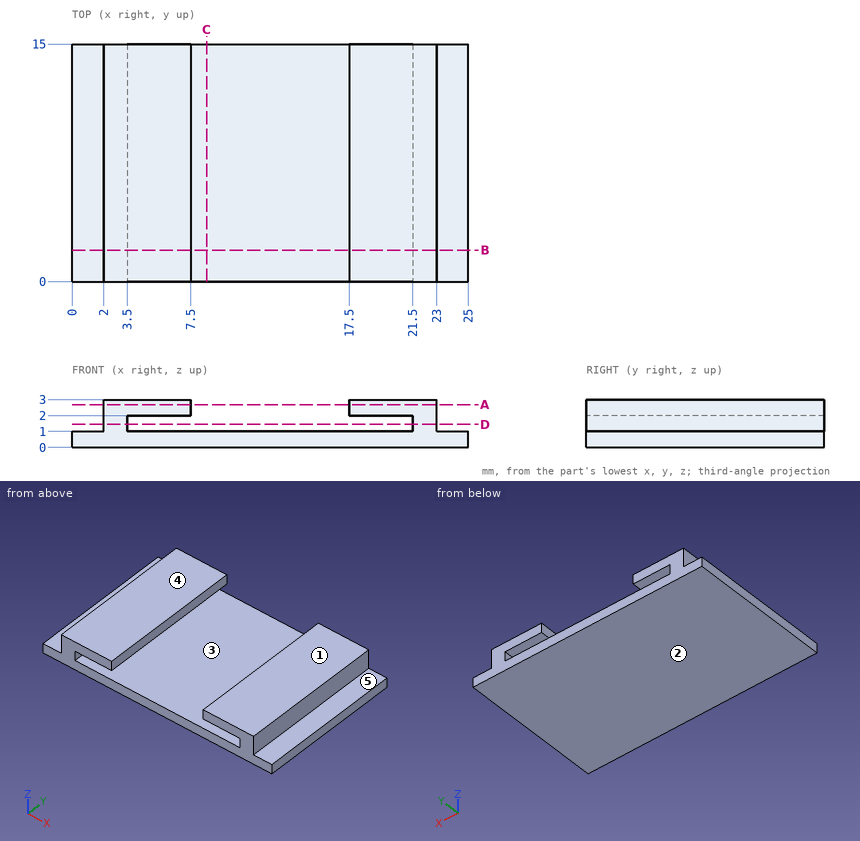
Drawing for the job (mm, zero at the part's lowest x, y, z). A direction names the side the tool comes from. Round coordinates to 2 decimals unless told otherwise and drop trailing zeros. Loops run counter-clockwise (first coordinate to the right, second up) from the corner with the lowest first, then second, coordinate; pieces in that order, holes last. Notation, with made-up numbers: (46.25, 8) - (51.25, 8) arc R9 ccw to (51.25, 17) - close; hole circle Ø9 at (86, 35). An arc over 180 degrees is marked (long way). Write each question's results on one line, items separated by ' | '.
(1) Mould opens along Z. For the marked faces 1, 2 and 3 say: released by +Z, released by -Z, zero draft, split by the parting line, or undercut.
Answer below:
face 1: released by +Z | face 2: released by -Z | face 3: undercut
(2) Pin check, flat tips, straight feed: pin 1 (6 mm diameter, centred on x = 11, y = 11, fed in from +Z); pin 2 (0.8 mm diameter, centred on y = 8.5, z = 1.5, fed in from -X); pin 3 (0.8 mm diameter, centred on y = 8.5, z = 1.5, fed in from +X). Stop position of each tip, or through.
Answer below:
pin 1: stops at z = 1 | pin 2: stops at x = 2 | pin 3: stops at x = 23
(3) Saw through at C-C, the plane x = 8.5. List the corners of the cut face in (y, z).
Answer below:
outline: (0, 0) - (15, 0) - (15, 1) - (0, 1) - close
(4) Saw through at A-A, the plane z = 2.7. List the corners of the cut face in (x, y).
Answer below:
outline: (2, 0) - (7.5, 0) - (7.5, 15) - (2, 15) - close; (17.5, 0) - (23, 0) - (23, 15) - (17.5, 15) - close
(5) Wall check: L1, parallel to X at y = 4.25, z = 1.55; L2, parallel to X at y = 8, z = 2.9; L3, parallel to Z at x = 7, y = 1.5. Give the ranges that are in metal, low to high.
Answer below:
L1: x = 2 to 3.5, 21.5 to 23 | L2: x = 2 to 7.5, 17.5 to 23 | L3: z = 0 to 1, 2 to 3
(6) Saw through at D-D, the plane z = 1.45. List the corners of the cut face in (x, y), then the cut area to 3 significant figures.
Answer below:
outline: (2, 0) - (3.5, 0) - (3.5, 15) - (2, 15) - close; (21.5, 0) - (23, 0) - (23, 15) - (21.5, 15) - close | area: 45.0 mm^2
(7) 3-axis set-ups, long thin cutter, end or side, ignore diameter. For the marked faces 4 and 5: which of +Z, -Z, +X, -X, +Y, -Y reach the whole face in a straight line?
Answer below:
face 4: +Z, +X, -X, +Y, -Y | face 5: +Z, +X, +Y, -Y
(8) Saw through at B-B, the plane y = 2. List the corners of the cut face in (x, z), then the cut area to 3 significant figures.
Answer below:
outline: (0, 0) - (25, 0) - (25, 1) - (23, 1) - (23, 3) - (17.5, 3) - (17.5, 2) - (21.5, 2) - (21.5, 1) - (3.5, 1) - (3.5, 2) - (7.5, 2) - (7.5, 3) - (2, 3) - (2, 1) - (0, 1) - close | area: 39.0 mm^2
